Read the model definition and answer for the solid it produces. Units are mm, in the model's axes. A direction names the side the tool comes from. Give positions to 0.01 mm unless a question says otherwise; leave off trailing zeros. Order: outer loops, then holes, each group sorted by start corner. A loop starts at its lowest first (then second) coordinate and runs counter-clockwise, first axis right, second up. Notation, with made-up numbers: (38.25, 55.25) - (95.25, 55.25) arc R30 cw to (95.25, 77.25) - close; hole circle Ø1 at (-19.75, 26). An arc over 180 degrees is marked (long way). Use a Markdown table: item, result. Add a question column.
1. A cutting plane is placed at D-D on y = 93.5. Determine the outline of the cut face in (x, z).
2. A cutting plane is placed at A-A on z = 0. State how many separate pieces and enclosed holes the cut face has, and give its area (3 significant figures).
3. Flat-ended cylindrical pins translate along their axes: P1, Ø3, axis at y = 26, z = 19.5, coming from the -X side; P2, Ø17.5, axis at x = -54.5, z = -3, coming from the -Y side; P3, Ø7.5, axis at y = 132.5, z = -50, coming from the -X side; P4, Ø18, axis at y = 65, z = 60, coming from the -X side. Find the tip coordinate at first contact, or state that the pin passes through.
4. Which of the six approach directions +Z, -Z, +X, -X, +Y, -Y give full straight-line access (tool end or side, diameter ignored) to faces 1 (the flat face through (-50, 57, 8)), 2 (the flat face through (22, 100, 21)), 3 (the flat face through (12, 135, -50))?
5. For a pull along X with two mould halves and no side action, classify faces 4 (the flat face through (-49, 37, 0)), 5 (the flat face through (8, 57, 50)), 6 (the cylindrical face through (12.932, 23.171, -5.362)) as released by +X, released by -X, zero draft, split by the parting line, or undercut.
6. Consider L1, parallel to Y at x = 60, z = -0.25; L2, parallel to Y at x = -4, z = -60; L3, parallel to Z at x = -41.5, y = 65. Determine where each line is inside the solid, lowest interval first.
```python
from build123d import *

# Parameters (mm, degrees)
SKETCH_1_R               = 55
EXTRUDE_1_DEPTH          = 150
SKETCH_2_R               = 30
CUT_EXTRUDE_1_DEPTH      = 100
SKETCH_3_R               = 48.25
CUT_EXTRUDE_2_DEPTH      = 50
SKETCH_4_R               = 60
SKETCH_4_R_2             = 40
CUT_EXTRUDE_1_2_DEPTH    = 90
EXTRUDE_START            = 30
SKETCH_6_W               = 16
SKETCH_6_H               = 53.194792051
EXTRUDE_3_DEPTH          = 50
EXTRUDE_START_2          = -30
SKETCH_10_W              = 16
SKETCH_10_H              = 53.194792051
EXTRUDE_4_DEPTH          = 50
SKETCH_11_W              = 16
SKETCH_11_H              = 53
EXTRUDE_6_DEPTH          = 50
SKETCH_12_W              = 16
SKETCH_12_H              = 53
EXTRUDE_7_DEPTH          = 50
FILLET_1_R               = 20
FILLET_2_R               = 20
FILLET_3_R               = 20
FILLET_4_R               = 20
CUT_EXTRUDE_4_DEPTH      = 40
CUT_EXTRUDE_4_DEPTH_BACK = 40
SKETCH_15_R              = 10
CUT_EXTRUDE_5_DEPTH      = 40
CUT_EXTRUDE_5_DEPTH_BACK = 40
SKETCH_16_R              = 10
SKETCH_17_W              = 24
SKETCH_17_H              = 14.571737585
CUT_EXTRUDE_6_DEPTH      = 87
SKETCH_18_R              = 34
SKETCH_18_R_2            = 14
EXTRUDE_1_2_DEPTH        = 47


with BuildPart() as part:
    # 草图1 → Extrude 1 (new body)
    with BuildSketch(Plane(origin=(0, 0, 0), x_dir=(1, 0, 0), z_dir=(0, 1, 0))):
        with Locations(Location((0, 0, 0), (0, 0, 270))):
            Circle(SKETCH_1_R)
    extrude(amount=EXTRUDE_1_DEPTH)

    # 草图2 → Cut-Extrude 1 (cut)
    with BuildSketch(Plane.XZ):
        with Locations(Location((0, 0, 0), (0, 0, 270))):
            Circle(SKETCH_2_R)
    extrude(amount=-CUT_EXTRUDE_1_DEPTH, mode=Mode.SUBTRACT)

    # 草图3 → 切除-拉伸2 (cut)
    with BuildSketch(Plane(origin=(0, 150, 0), x_dir=(1, 0, 0), z_dir=(0, 1, 0))):
        with Locations(Location((0, 0, 0), (0, 0, 270))):
            Circle(SKETCH_3_R)
    extrude(amount=-CUT_EXTRUDE_2_DEPTH, mode=Mode.SUBTRACT)

    # 草图4 → Cut-Extrude 1 2 (cut)
    with BuildSketch(Plane.XZ):
        Circle(SKETCH_4_R)
        Circle(SKETCH_4_R_2, mode=Mode.SUBTRACT)
    extrude(amount=-CUT_EXTRUDE_1_2_DEPTH, mode=Mode.SUBTRACT)

    # 草图11 → 凸台-拉伸6 (add)
    with BuildSketch(Plane(origin=(0, 0, 0), x_dir=(0, 0, -1), z_dir=(1, 0, 0)).offset(EXTRUDE_START)):
        with Locations((0, 63.5)):
            Rectangle(SKETCH_11_W, SKETCH_11_H)
    extrude(amount=EXTRUDE_6_DEPTH)

    # 草图12 → 凸台-拉伸7 (add)
    with BuildSketch(Plane(origin=(0, 0, 0), x_dir=(0, 0, -1), z_dir=(1, 0, 0)).offset(EXTRUDE_START_2)):
        with Locations((0, 63.5)):
            Rectangle(SKETCH_12_W, SKETCH_12_H)
    extrude(amount=-EXTRUDE_7_DEPTH)

    # 圆角1
    fillet_1_edges = [part.edges().sort_by_distance(p)[0] for p in [
        (-80, 90, 0),
        (-80, 37, 0),
    ]]
    fillet(fillet_1_edges, radius=FILLET_1_R)

    # 圆角3
    fillet_3_edges = [part.edges().sort_by_distance(p)[0] for p in [
        (80, 37, 0),
        (80, 90, 0),
    ]]
    fillet(fillet_3_edges, radius=FILLET_3_R)

    # 草图15 → 切除-拉伸4 (cut, two sides: drawn at the far end of the back side and taken through both)
    with BuildSketch(Plane.XY.offset(-CUT_EXTRUDE_4_DEPTH_BACK)):
        with Locations(Location((60, 65, 0), (0, 0, 180))):
            Circle(SKETCH_15_R)
        with Locations(Location((-60, 65, 0), (0, 0, 180))):
            Circle(SKETCH_15_R)
    extrude(amount=CUT_EXTRUDE_4_DEPTH + CUT_EXTRUDE_4_DEPTH_BACK, mode=Mode.SUBTRACT)

    # 草图17 → 切除-拉伸6 (cut)
    with BuildSketch(Plane.XY):
        with Locations((0, 134.985868793)):
            Rectangle(SKETCH_17_W, SKETCH_17_H)
    extrude(amount=-CUT_EXTRUDE_6_DEPTH, mode=Mode.SUBTRACT)



with BuildPart() as body_2:
    # 草图6 → 凸台-拉伸3 (new body)
    with BuildSketch(Plane.XY.offset(EXTRUDE_START)):
        with Locations((0, 63.37627806)):
            Rectangle(SKETCH_6_W, SKETCH_6_H)
    extrude(amount=EXTRUDE_3_DEPTH)

    # 圆角4
    fillet_4_edges = [body_2.edges().sort_by_distance(p)[0] for p in [
        (0, 36.778882035, 80),
        (0, 89.973674086, 80),
    ]]
    fillet(fillet_4_edges, radius=FILLET_4_R)


with BuildPart() as body_3:
    # 草图10 → 凸台-拉伸4 (new body)
    with BuildSketch(Plane.XY.offset(EXTRUDE_START_2)):
        with Locations((0, 63.37627806)):
            Rectangle(SKETCH_10_W, SKETCH_10_H)
    extrude(amount=-EXTRUDE_4_DEPTH)

    # 圆角2
    fillet_2_edges = [body_3.edges().sort_by_distance(p)[0] for p in [
        (0, 89.973674086, -80),
        (0, 36.778882035, -80),
    ]]
    fillet(fillet_2_edges, radius=FILLET_2_R)


with BuildPart() as cut_extrude_5_tool:
    # 草图16 → 切除-拉伸5 (new, two sides: drawn at the far end of the back side and taken through both)
    with BuildSketch(Plane(origin=(0, 0, 0), x_dir=(0, 0, -1), z_dir=(1, 0, 0)).offset(-CUT_EXTRUDE_5_DEPTH_BACK)):
        with Locations(Location((60, 65, 0), (0, 0, 180))):
            Circle(SKETCH_16_R)
        with Locations(Location((-60, 65, 0), (0, 0, 270))):
            Circle(SKETCH_16_R)
    extrude(amount=CUT_EXTRUDE_5_DEPTH + CUT_EXTRUDE_5_DEPTH_BACK)


with BuildPart() as body_2_1:
    add(body_2.part)

    # 切除-拉伸5: cut by cut_extrude_5_tool
    add(cut_extrude_5_tool.part, mode=Mode.SUBTRACT)


with BuildPart() as body_3_1:
    add(body_3.part)

    # 切除-拉伸5: cut by cut_extrude_5_tool
    add(cut_extrude_5_tool.part, mode=Mode.SUBTRACT)


with BuildPart() as part_1:
    add(part.part)

    add(body_2_1.part)  # Extrude 1 2 merges body 2

    add(body_3_1.part)  # Extrude 1 2 merges body 3
    # 草图18 → Extrude 1 2 (add)
    with BuildSketch(Plane.XZ):
        Circle(SKETCH_18_R)
        Circle(SKETCH_18_R_2, mode=Mode.SUBTRACT)
    extrude(amount=-EXTRUDE_1_2_DEPTH)

    # 倒角1: read off the stored shape, not the designer's step
    # 倒角1 outline → 倒角1 (revolve, cut)
    with BuildSketch(Plane.XY):
        Polygon((40, 36.5), (14.442424855, 0), (40, 0), align=None)
    revolve(axis=Axis((0, 0, 0), (0, 1, 0)), mode=Mode.SUBTRACT)


solid = part_1.part
```
Output values:
| question | item | result |
|---|---|---|
| 1 | outline | circle Ø110 at (0, 0); hole circle Ø60 at (0, 0) |
| 2 | separate pieces | 2 |
| 2 | enclosed holes | 2 |
| 2 | area | 6,810 mm² |
| 3 | P1 | x = -27.85 |
| 3 | P2 | y = 37 |
| 3 | P3 | x = -29.76 |
| 3 | P4 | through |
| 4 | face 1 | +Z, -X, -Y |
| 4 | face 2 | +Y |
| 4 | face 3 | -Z |
| 5 | face 4 | zero draft |
| 5 | face 5 | released by +X |
| 5 | face 6 | undercut |
| 6 | L1 | 37 to 55, 75 to 90 |
| 6 | L2 | 36.78 to 55, 75 to 89.97 |
| 6 | L3 | -8 to 8 |
